```python
from build123d import *

# Parameters (mm, degrees)
F2_R     = 7.1
F2_R_2   = 5.5
F3_DEPTH = 20
F1_R     = 7.1
F1_R_2   = 5.5
F4_DEPTH = 20
F0_R     = 7.1
F0_R_2   = 5.5
F5_DEPTH = 20


with BuildPart() as f3:
    # F2 (on Right) → F3 (new body)
    with BuildSketch(Plane.YZ):
        Circle(F2_R)
        Circle(F2_R_2, mode=Mode.SUBTRACT)
    extrude(amount=F3_DEPTH)

    # F1 (on Front) → F4 (join)
    with BuildSketch(Plane.XZ):
        Circle(F1_R)
        Circle(F1_R_2, mode=Mode.SUBTRACT)
    extrude(amount=F4_DEPTH)

    # F0 (on Top) → F5 (join)
    with BuildSketch(Plane.XY):
        Circle(F0_R)
        Circle(F0_R_2, mode=Mode.SUBTRACT)
    extrude(amount=F5_DEPTH)


solid = f3.part
```
CAD build for the part. Positions are in the model's coordinates, mm. A direction names the side the tool comes from. Round coordinates to 2 decimals unless told otherwise and drop trailing zeros. Write each loop counter-clockwise with the first axis right and the second up, starting at its lowest first coordinate (ties: lowest second). Pieces come first, ordered by that corner, then holes.
Item 1: Mould opens along Y. For faces 1 (the cylindrical face through (-5.634, -12.082, -4.32)), 2 (the cylindrical face through (1.49, -3.85, 3.93)), 3 (the cylindrical face through (-5.23, 4.8, 12.08)) say: released by +Y, released by -Y, zero draft, split by the parting line, or undercut.
Filled in:
face 1: zero draft
face 2: undercut
face 3: split by the parting line
Item 2: Band-saw the part on A-A on y = 1.75. Write the cut outline in (x, z).
Filled in:
outline: (-6.88, 0) - (-5.21, 0) - (-5.21, 20) - (-6.88, 20) - close; (0, -6.88) - (20, -6.88) - (20, -5.21) - (0, -5.21) - close; (0, 5.21) - (5.21, 5.21) - (5.21, 0) - (6.88, 0) - (6.88, 5.21) - (20, 5.21) - (20, 6.88) - (6.88, 6.88) - (6.88, 20) - (5.21, 20) - (5.21, 6.88) - (0, 6.88) - close
Item 3: Drill centre lines: L1, parallel to Y at x = 15.5, z = 0; L2, parallel to Z at x = 4, y = 4.75. Where is each one in solid material? Low to high.
Filled in:
L1: y = -7.1 to -5.5, 5.5 to 7.1
L2: z = -5.28 to -2.77, 0 to 20
Item 4: Band-saw the part on C-C on x = 10. Write the cut outline in (y, z), then the cut area to 3 significant figures.
Filled in:
outline: circle Ø14.2 at (0, 0); hole circle Ø11 at (0, 0)
area: 63.3 mm2
Item 5: Drop flat-ended pins along their axis: pin 1 Ø5 at (x, z) = (7, 9.5) entering from +Y; pin 2 Ø8 at (y, z) = (-14, 10.5) entering from -X; pin 3 Ø3 at (x, z) = (3, 3) entering from +Y. Give the stop position or say it passes through.
Filled in:
pin 1: stops at y = 5.49
pin 2: stops at x = -2.86
pin 3: stops at y = 6.94
Item 6: Band-saw the part on B-B on z = -0.75. Write the cut outline in (x, y).
Filled in:
outline: (-7.06, -20) - (-5.45, -20) - (-5.45, 0) - (-7.06, 0) - close; (0, -7.06) - (5.45, -7.06) - (5.45, -20) - (7.06, -20) - (7.06, -7.06) - (20, -7.06) - (20, -5.45) - (7.06, -5.45) - (7.06, 0) - (5.45, 0) - (5.45, -5.45) - (0, -5.45) - close; (0, 5.45) - (20, 5.45) - (20, 7.06) - (0, 7.06) - close
Item 7: Tool access for faces 4 (the cylindrical face through (5.01, -5.03, 0.86)), 5 (the flat face through (-4, 4, 0)), 6 (the cylindrical face through (12.08, 5.08, -2.11)), 7 (the cylindrical face through (-4.05, 3.72, 12.08)): list every direction of +Z, -Z, +X, -X, +Y, -Y with a clear straight run to the whole face (end or side of a thin tool).
Filled in:
face 4: none
face 5: -Z, -X, +Y
face 6: +X
face 7: +Z
